from build123d import *

# Parameters (mm, degrees)
F0_W          = 16
F0_H          = 30
F1_DEPTH      = 142.5
F1_DEPTH_BACK = 142.5
F2_W          = 16
F2_H          = 30
F3_DEPTH      = 17.5
F4_R          = 2


# Not quite as in the source:
# - a pattern or mirror of a feature is missing from the dataset's text; its kind, count and spacing are read off the source's solid


with BuildPart() as f1:
    # F0 (on Front) → F1 (new body, two sides)
    with BuildSketch(Plane.XZ) as f1_sk:
        Rectangle(F0_W, F0_H)
    extrude(amount=F1_DEPTH)
    extrude(f1_sk.sketch, amount=-F1_DEPTH_BACK)

    # F2 (on face) → F3 (cut)
    with BuildSketch(Plane.XZ.offset(142.5)):
        Rectangle(F2_W, F2_H)
        with BuildLine():
            ThreePointArc((5, -7.5), (0, -12.5), (-5, -7.5))
            Line((-5, -7.5), (-5, 7.5))
            ThreePointArc((-5, 7.5), (0, 12.5), (5, 7.5))
            Line((5, 7.5), (5, -7.5))
        make_face(mode=Mode.SUBTRACT)
    f3 = extrude(amount=-F3_DEPTH, mode=Mode.SUBTRACT)

    # F3_copies: F3 across plane
    add(f3.mirror(Plane.ZX), mode=Mode.SUBTRACT)

    # F4
    f4_edges = [f1.edges().sort_by_distance(p)[0] for p in [
        (-8, 0, 15),
        (8, 0, 15),
        (8, 0, -15),
        (-8, 0, -15),
    ]]
    fillet(f4_edges, radius=F4_R)


solid = f1.part
Design review of the part built by this model. Coordinates are the model's own, in mm. A direction names the side the tool comes from. Give positions to 0.01 mm unless a question says otherwise; leave off trailing zeros. Order: outer loops, then holes, each group sorted by start corner. A loop starts at its lowest first (then second) coordinate and runs counter-clockwise, first axis right, second up. Notation, with made-up numbers: (-15, -5) - (27, -5) arc R34 ccw to (27, 34) - close; hole circle Ø9 at (80, 16.25). An arc over 180 degrees is marked (long way). Write item = value, one per line. Start each with the question number.
Q1. We need section B-B on x = 0. State the section outline as (y, z) points, plus the area to 4 significant figures.
Q2. To check wall thickness, follow L1, parallel to Y at x = 3.75, z = 12.25; L2, parallel to Z at x = 6.25, y = 96.5; L3, parallel to X at y = -70.5, z = 13.25. State the ranges of each line that lie inside material, in increasing order. Write a range as from..to.
Q3. We need section A-A on z = 4.5. State the section outline as (x, y) points, plus the area to 3 significant figures.
Q4. Tool access review of faces 1 (the face through (5, 134, 0)), 2 (the face through (-5, 134, 0)), 3 (the face through (-0.1, 133.9, 12.5)), 4 (the face through (0.1, -133.9, -12.5)): name each direction out of +Z, -Z, +X, -X, +Y, -Y from which nothing blocks a thin tool from reaching the whole face with its end or side.
Q5. Clearance check with flat-ended pins moving along their axes: pin 1 Ø16.5 at (y, z) = (-131.5, 0.5) entering from -X; pin 2 Ø12 at (y, z) = (-134, -3.5) entering from +X; pin 3 Ø12 at (y, z) = (134, 0.5) entering from -X. State where each tip first meets the part, or that it passes through.
Working result:
q1.outline = (-142.5, -12.5) - (-125, -12.5) - (-125, -15) - (125, -15) - (125, -12.5) - (142.5, -12.5) - (142.5, 12.5) - (125, 12.5) - (125, 15) - (-125, 15) - (-125, 12.5) - (-142.5, 12.5) - close
q1.area = 8,375 mm²
q2.L1 = -125..125
q2.L2 = -14.98..14.98
q2.L3 = -7.98..7.98
q3.outline = (-8, -125) - (-5, -125) - (-5, -142.5) - (5, -142.5) - (5, -125) - (8, -125) - (8, 125) - (5, 125) - (5, 142.5) - (-5, 142.5) - (-5, 125) - (-8, 125) - close
q3.area = 4,350 mm²
q4.face_1 = +Z, -Z, +X, +Y
q4.face_2 = +Z, -Z, -X, +Y
q4.face_3 = +Z, +Y
q4.face_4 = -Z, -Y
q5.pin_1 = -8
q5.pin_2 = 5
q5.pin_3 = -5
